from build123d import *

# Parameters (mm, degrees)
BOSS_EXTRUDE1_DEPTH            = 444.55
FILLET1_R                      = 1.5875
CUT_EXTRUDE1_DEPTH             = 452.571262372
CUT_EXTRUDE1_DEPTH_BACK        = 452.571262372
F_7_9_7_9_DIAMETER_HOLE1_D     = 7.9
F_7_9_7_9_DIAMETER_HOLE1_DEPTH = 15
F_7_9_7_9_DIAMETER_HOLE1_TIP   = 2.373399445


with BuildPart() as part:
    # Sketch1 → Boss-Extrude1 (new, symmetric)
    with BuildSketch(Plane.XY):
        Polygon((0, 77), (0, 0), (4.05, 0), (4.05, 9.525), (19.05, 9.525), (19.05, 70), (4.05, 70), (4.05, 77), align=None)
    extrude(amount=BOSS_EXTRUDE1_DEPTH, both=True)

    # Fillet1
    fillet1_edges = [part.edges().sort_by_distance(p)[0] for p in [
        (0, 0, 0),
        (0, 77, 0),
    ]]
    fillet(fillet1_edges, radius=FILLET1_R)

    # Sketch2 → Cut-Extrude1 (cut, two sides: drawn at the far end of the back side and taken through both)
    with BuildSketch(Plane(origin=(0, 77, 0), x_dir=(1, 0, 0), z_dir=(0, 1, 0)).offset(-CUT_EXTRUDE1_DEPTH_BACK)):
        Polygon((0, -444.55), (19.05, -425.5), (19.05, -444.55), align=None)
        Polygon((0, 444.55), (19.05, 425.5), (19.05, 444.55), align=None)
    extrude(amount=CUT_EXTRUDE1_DEPTH + CUT_EXTRUDE1_DEPTH_BACK, mode=Mode.SUBTRACT)

    # Ø7.9 (7.9) Diameter Hole1
    with Locations(Plane(origin=(0, 9.525, 0), x_dir=(-1, 0, 0), z_dir=(0, -1, 0))):
        with Locations((-11.55, -410.5), (-11.55, 410.5), (-11.55, 0)):
            Hole(F_7_9_7_9_DIAMETER_HOLE1_D / 2, depth=F_7_9_7_9_DIAMETER_HOLE1_DEPTH)
            with Locations((0, 0, -(F_7_9_7_9_DIAMETER_HOLE1_DEPTH + F_7_9_7_9_DIAMETER_HOLE1_TIP / 2))):  # 118° drill point
                Cone(0, F_7_9_7_9_DIAMETER_HOLE1_D / 2, F_7_9_7_9_DIAMETER_HOLE1_TIP, mode=Mode.SUBTRACT)


solid = part.part
The model under review builds one solid part; all positions refer to its coordinate system, in mm. A direction names the side the tool comes from. Coordinates: 2 decimals unless noted, no trailing zeros. Loops run counter-clockwise (first coordinate to the right, second up) from the corner with the lowest first, then second, coordinate; pieces in that order, holes last. Notation, with made-up numbers: M -36.75,-3.75 L 13.25,-3.75 A20 ccw 13.25,18.25 Z; hole C -23.75,-34 d6. An arc over 180 degrees is marked long. Put each result on its own line as item: value. Start each with the question number.
Q1. Add section B-B (y = 55.5). Write out the cut boundary in (x, z), and give its area (3 significant figures).
Q2. Clearance check with flat-ended pins moving along their axes: pin 1 (8 mm diameter, centred on x = 11, y = 66, fed in from +Z); pin 2 (10.5 mm diameter, centred on x = 11.55, z = -410.5, fed in from -Y) (3 decimals); pin 3 (7.5 mm diameter, centred on y = 4.5, z = -219, fed in from +X). State where each tip first meets the part, or that it passes through.
Q3. Wall thickness on line 1 (X direction, y = 16.25, z = 410.5); line 2 (Z direction, x = 11.55, y = 16); line 3 (Z direction, x = 1.5, y = 62.5): over which ranges is each line inside the solid? List them lowest first.
Q4. For faces 1 (the flat face through (9.39, 37.96, -435.16)), 2 (the flat face through (11, 9.525, 6)), 3 (the flat face through (12, 70, 6)), list the 3-axis set-ups (+Z, -Z, +X, -X, +Y, -Y) from which the entire face can be reached by the end or side of a thin tool; tool diameter is ignored.
Answers:
1. outline: M 0,-444.55 L 19.05,-425.5 L 19.05,425.5 L 0,444.55 Z
1. area: 16,600 mm^2
2. pin 1: stops at z = 437.55
2. pin 2: stops at y = 9.525
2. pin 3: stops at x = 4.05
3. line 1: x = 0 to 7.6, 15.5 to 19.05
3. line 2: z = -433 to -414.45, -406.55 to -3.95, 3.95 to 406.55, 414.45 to 433
3. line 3: z = -443.05 to 443.05
4. face 1: -Z, +X, +Y, -Y
4. face 2: +Z, -Z, +X, -Y
4. face 3: +Z, -Z, +X, +Y
